The model under review builds one solid part; all positions refer to its coordinate system, in mm. Round coordinates to 2 decimals unless told otherwise and drop trailing zeros. Write each loop counter-clockwise with the first axis right and the second up, starting at its lowest first coordinate (ties: lowest second). Pieces come first, ordered by that corner, then holes. Notation, with made-up numbers: M 61.25,-5.75 L 120.25,-5.75 A14 cw 120.25,13.25 Z; hole C 41,11 d2. An arc over 180 degrees is marked long. Write item = value, one per line. Start each with the question number.
Item 1: Take a section at B-B, the plane x = -10. Give the boundary of the cut face in (y, z), plus the area to 3 significant figures.
Item 2: To check wall thickness, follow line 1 along X through (y, z) = (-4.75, 1); line 2 along Y through (x, z) = (-15, -11.5); line 3 along Y through (x, z) = (3.5, -4.75). State the ranges of each line that lie inside material, in increasing order.
Item 3: Take a section at A-A, the plane z = -1.5. Give the boundary of the cut face in (x, y), plus the area to 3 significant figures.
Item 4: Take a section at C-C, the plane y = -21.5. Give the boundary of the cut face in (x, z).
from build123d import *

# Parameters (mm, degrees)
F0_W     = 63.5
F0_H     = 25.4
F1_DEPTH = 25.4
F2_R     = 5.08
F3_SIZE2 = 12.7
F3_SIZE  = 7.62


with BuildPart() as f1:
    # F0 (on Front) → F1 (new body)
    with BuildSketch(Plane.XZ):
        Rectangle(F0_W, F0_H)
    extrude(amount=F1_DEPTH)

    # F2
    f2_edges = [f1.edges().sort_by_distance(p)[0] for p in [
        (31.75, 0, 0),
    ]]
    fillet(f2_edges, radius=F2_R)

    # F3
    f3_edges = [f1.edges().sort_by_distance(p)[0] for p in [
        (0, -25.4, -12.7),
    ]]
    chamfer(f3_edges, length=F3_SIZE, length2=F3_SIZE2)


solid = f1.part
Response values:
q1.outline = M -25.4,0 L -17.78,-12.7 L 0,-12.7 L 0,12.7 L -25.4,12.7 Z
q1.area = 597 mm2
q2.line_1 = -31.75 to 31.74
q2.line_2 = -18.5 to 0
q2.line_3 = -22.55 to 0
q3.outline = M -31.75,-24.5 L 31.75,-24.5 L 31.75,-5.08 A5.08 ccw 26.67,0 L -31.75,0 Z
q3.area = 1,550 mm2
q4.outline = M -31.75,-6.5 L 31.75,-6.5 L 31.75,12.7 L -31.75,12.7 Z
